Work out the finished part from the listing and answer in its coordinate system (mm). Face numbers are marked on the shaded views. A direction names the side the tool comes from. Give positions to 0.01 mm unless a question says otherwise; leave off trailing zeros. Order: outer loops, then holes, each group sorted by start corner. A loop starts at its lowest first (then second) coordinate and runs counter-clockwise, first axis right, second up. Notation, with made-up numbers: (58, 72.25) - (95, 72.25) arc R15 cw to (95, 83.25) - close; hole circle Ø6 at (17.25, 82). An arc over 180 degrees is marked (long way). Put each result on its own line as item: value.
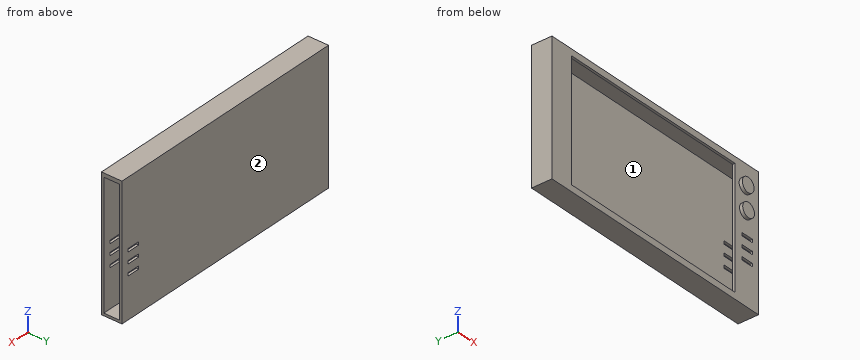
```python
from build123d import *

# Parameters (mm, degrees)
F0_W      = 158
F0_H      = 83
F1_DEPTH  = 13
F2_W      = 125
F2_H      = 75
F3_DEPTH  = 10
F4_W      = 10
F4_H      = 79
F5_DEPTH  = 157
F6_R      = 4.5
F7_DEPTH  = 2
F8_R      = 4.5
F9_DEPTH  = 2
F10_W     = 8
F10_H     = 2
F11_DEPTH = 25


with BuildPart() as f1:
    # F0 (on Front) → F1 (new body)
    with BuildSketch(Plane.XZ):
        with Locations((79, 41.5)):
            Rectangle(F0_W, F0_H)
    extrude(amount=F1_DEPTH)

    # F2 (on face) → F3 (cut)
    with BuildSketch(Plane.XZ.offset(13)):
        with Locations((77.5, 41.5)):
            Rectangle(F2_W, F2_H)
    extrude(amount=-F3_DEPTH, mode=Mode.SUBTRACT)

    # F4 (on face) → F5 (cut)
    with BuildSketch(Plane.YZ.offset(158)):
        with Locations((-6.5, 41.0799)):
            Rectangle(F4_W, F4_H)
    extrude(amount=-F5_DEPTH, mode=Mode.SUBTRACT)

    # F6 (on face) → F7 (join)
    with BuildSketch(Plane.XZ.offset(13)):
        with Locations((147.664174, 69.502406)):
            Circle(F6_R)
    extrude(amount=F7_DEPTH)

    # F8 (on face) → F9 (join)
    with BuildSketch(Plane.XZ.offset(13)):
        with Locations((147.959903, 55.012029)):
            Circle(F8_R)
    extrude(amount=F9_DEPTH)

    # F10 (on face) → F11 (cut)
    with BuildSketch(Plane.XZ.offset(13)):
        with Locations((149.298406, 40.5)):
            Rectangle(F10_W, F10_H)
        with Locations((149.298406, 33.5)):
            Rectangle(F10_W, F10_H)
        with Locations((149.298406, 26.5)):
            Rectangle(F10_W, F10_H)
    extrude(amount=-F11_DEPTH, mode=Mode.SUBTRACT)


solid = f1.part
```
(1) Straight lines are drawn through the part: line 1 (Z direction, x = 87.5, y = -5.5); line 2 (Y direction, x = 9, z = 38.5); line 3 (X direction, y = -4.5, z = 73.5). For each, find the intervals that lie inside material, in ascending order.
Geometry check:
line 1: z = 0 to 1.58, 80.58 to 83
line 2: y = -13 to -11.5, -1.5 to 0
line 3: x = 0 to 1
(2) Section A-A, the plane z = 45 is taken. Write down the section's boundary in (x, y), then the cut area to 4 significant figures.
Geometry check:
outline: (0, -13) - (15, -13) - (15, -11.5) - (1, -11.5) - (1, -1.5) - (158, -1.5) - (158, 0) - (0, 0) - close; (140, -13) - (158, -13) - (158, -11.5) - (140, -11.5) - close
area: 296.5 mm²
(3) Section C-C, the plane x = 74.5 is taken. Write down the section's boundary in (y, z).
Geometry check:
outline: (-13, 0) - (0, 0) - (0, 83) - (-13, 83) - (-13, 79) - (-11.5, 79) - (-11.5, 80.58) - (-1.5, 80.58) - (-1.5, 1.58) - (-11.5, 1.58) - (-11.5, 4) - (-13, 4) - close
(4) Section B-B, the plane y = -10 is taken. Write down the section's boundary in (x, z), then the cut area to 3 significant figures.
Geometry check:
outline: (0, 0) - (158, 0) - (158, 1.58) - (1, 1.58) - (1, 80.58) - (158, 80.58) - (158, 83) - (0, 83) - close
area: 711 mm²
(5) Given pin 1 (8 mm diameter, centred on y = -7, z = 59, fed in from +X), flat-ended and moving along its own axis, determine where the tip first touches the part or whether it passes through.
Geometry check:
pin 1: stops at x = 1
(6) A tool of negligible diameter and unlimited length cuts with its end or side. For the marked faces 1 and 2, from which of +Z, -Z, +X, -X, +Y, -Y can it reach the whole face along a straight path? Write none if from no direction.
Geometry check:
face 1: +X
face 2: +Z, -Z, +X, -X, +Y
